from build123d import *

# Parameters (mm, degrees)
SKETCH1_R                = 36.576
SKETCH1_R_2              = 28.6004
EXTRUDE1_DEPTH           = 7.9248
CHAMFER1_SIZE            = 0.519176
CHAMFER2_SIZE            = 1.1176
CUT_EXTRUDE1_DEPTH       = 8.9248
FILLET1_R                = 0.4064
CIRPATTERN1_COUNT        = 4
FILLET1_OF_CIRPATTERN1_R = 0.4064


with BuildPart() as part:
    # Sketch1 → Extrude1 (new body)
    with BuildSketch(Plane.XY):
        Circle(SKETCH1_R)
        Circle(SKETCH1_R_2, mode=Mode.SUBTRACT)
    extrude(amount=EXTRUDE1_DEPTH)

    # Chamfer1
    chamfer1_edges = [part.edges().sort_by_distance(p)[0] for p in [
        (-36.576, 0, 0),
        (-36.576, 0, 7.9248),
    ]]
    chamfer(chamfer1_edges, length=CHAMFER1_SIZE)

    # Chamfer2
    chamfer2_edges = [part.edges().sort_by_distance(p)[0] for p in [
        (-28.6004, 0, 0),
        (-28.6004, 0, 7.9248),
    ]]
    chamfer(chamfer2_edges, length=CHAMFER2_SIZE)

    # Sketch2 → Cut-Extrude1 (cut, through all)
    with BuildSketch(Plane.XY.offset(7.9248)):
        with BuildLine():
            Line((23.520447327, 28.010575388), (21.750180325, 26.240308386))
            Line((21.750180325, 26.240308386), (26.240308386, 21.750180325))
            Line((26.240308386, 21.750180325), (28.010575388, 23.520447327))
            ThreePointArc((28.010575388, 23.520447327), (25.863137629, 25.863137629), (23.520447327, 28.010575388))
        make_face()
    cut_extrude1 = extrude(amount=-CUT_EXTRUDE1_DEPTH, mode=Mode.SUBTRACT)

    # Fillet1
    fillet1_edges = [part.edges().sort_by_distance(p)[0] for p in [
        (26.240308386, 21.750180325, 3.9624),
        (21.750180325, 26.240308386, 3.9624),
    ]]
    fillet(fillet1_edges, radius=FILLET1_R)

    # CirPattern1: Cut-Extrude1 ×4 about axis
    cirpattern1_axis = Axis((0, 0, 0), (0, 0, 1))
    for i in range(1, CIRPATTERN1_COUNT):
        add(cut_extrude1.rotate(cirpattern1_axis, i * 360 / CIRPATTERN1_COUNT), mode=Mode.SUBTRACT)

    # Fillet1 of CirPattern1
    fillet1_of_cirpattern1_edges = [part.edges().sort_by_distance(p)[0] for p in [
        (-21.750180325, 26.240308386, 3.9624),
        (-26.240308386, 21.750180325, 3.9624),
        (-26.240308386, -21.750180325, 3.9624),
        (-21.750180325, -26.240308386, 3.9624),
        (21.750180325, -26.240308386, 3.9624),
        (26.240308386, -21.750180325, 3.9624),
    ]]
    fillet(fillet1_of_cirpattern1_edges, radius=FILLET1_OF_CIRPATTERN1_R)


solid = part.part
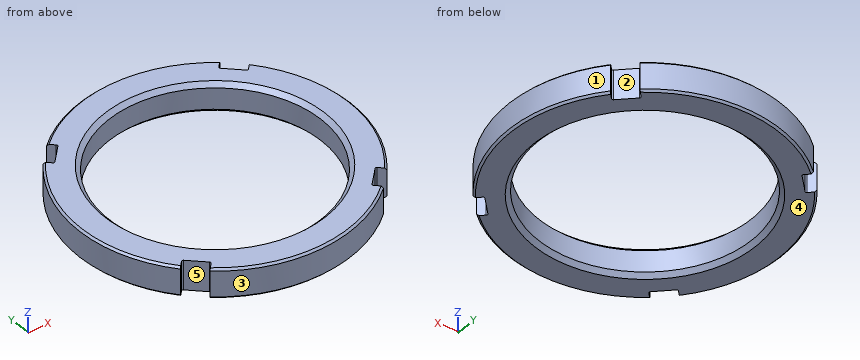
Verification items for the finished model (mm, model axes). Face numbers are marked on the shaded views. A direction names the side the tool comes from. Coordinates: 2 decimals unless noted, no trailing zeros. Write each loop counter-clockwise with the first axis right and the second up, starting at its lowest first coordinate (ties: lowest second). Pieces come first, ordered by that corner, then holes. Notation, with made-up numbers: (23, 66) -> (79, 66) arc R18 ccw to (79, 72) -> close; hole circle Ø9 at (32.25, 60.5). An arc over 180 degrees is marked (long way). One line per item, written item: value. Start each with the question number.
Q1. Cross-section at C-C on z = 4.75. Enter the section's corners in (x, y).
Q2. Access from +Z, -Z, +X, -X, +Y, -Y to the whole of each face (thin tool, end or side, straight path). Record for the marked faces 1 and 2.
Q3. Cross-section at A-A on y = 0. Enter the section's corners in (x, z).
Q4. Mould release check, pull along Y, two halves, no side actions. Record for the marked faces 3, 4 and 5: pulls with the +Y half, pulls with the -Y half, needs draft (parallel to the pull), parting line crosses it, or undercut.
Q5. Thickness scan on L1, parallel to X at y = -1, z = 5.25; L2, parallel to Y at x = -22.5, z = 5.5; L3, parallel to Y at x = 0, z = 3.2. Record the ranges inside material, lowest first. Write a range as from..to.
Q6. Go/stop test with flat-tipped pins: P1, Ø1.5, axis at y = -11, z = 6, coming from the -X side; P2, Ø4, axis at x = 16.5, z = 4.5, coming from the -Y side; P3, Ø1, axis at x = 14, z = 4.5, coming from the +Y side. Record where each tip stops, or that it passes through.
Checked values:
1. outline: (-28.01, -23.52) -> (-26.53, -22.04) arc R0.41 cw to (-25.95, -22.04) -> (-22.04, -25.95) arc R0.41 cw to (-22.04, -26.53) -> (-23.52, -28.01) arc R36.58 ccw to (23.52, -28.01) -> (22.04, -26.53) arc R0.41 cw to (22.04, -25.95) -> (25.95, -22.04) arc R0.41 cw to (26.53, -22.04) -> (28.01, -23.52) arc R36.58 ccw to (28.01, 23.52) -> (26.53, 22.04) arc R0.41 cw to (25.95, 22.04) -> (22.04, 25.95) arc R0.41 cw to (22.04, 26.53) -> (23.52, 28.01) arc R36.58 ccw to (-23.52, 28.01) -> (-22.04, 26.53) arc R0.41 cw to (-22.04, 25.95) -> (-25.95, 22.04) arc R0.41 cw to (-26.53, 22.04) -> (-28.01, 23.52) arc R36.58 ccw to start; hole circle Ø57.2 at (0, 0)
2. face 1: +Z, -Z, +X
2. face 2: +Z, -Z
3. outline: (-36.58, 0.52) -> (-36.06, 0) -> (-29.72, 0) -> (-28.6, 1.12) -> (-28.6, 6.81) -> (-29.72, 7.92) -> (-36.06, 7.92) -> (-36.58, 7.41) -> close; (28.6, 1.12) -> (29.72, 0) -> (36.06, 0) -> (36.58, 0.52) -> (36.58, 7.41) -> (36.06, 7.92) -> (29.72, 7.92) -> (28.6, 6.81) -> close
4. face 3: pulls with the -Y half
4. face 4: needs draft
4. face 5: undercut
5. L1: x = -36.56..-28.58, 28.58..36.56
5. L2: y = -28.84..-26.99, -25.49..-17.66, 17.66..25.49, 26.99..28.84
5. L3: y = -36.58..-28.6, 28.6..36.58
6. P1: stops at x = -35.11
6. P2: stops at y = -33.58
6. P3: stops at y = 33.99
